from build123d import *

# Parameters (mm, degrees)
SK_BODY_W                     = 46.51
SK_BODY_H                     = 11.1
BODY_DEPTH                    = 8.4
SK_FLANGE_EARS_W              = 4.8
SK_FLANGE_EARS_H              = 5.6
FLANGE_EARS_DEPTH             = 6
SK_NOSE_W                     = 46.51
SK_NOSE_H                     = 7
NOSE_DEPTH                    = 7.2
FLANGE_SCREW_HOLES_DEPTH      = 32.081232681
FLANGE_SCREW_HOLES_DEPTH_BACK = 32.081232681
SK_FLANGE_SCREW_HOLES_R       = 1.35
SK_WIRE_ENTRIES_W             = 2.6
SK_WIRE_ENTRIES_H             = 2.8
WIRE_ENTRIES_DEPTH            = 6
SK_CONTACT_OPENINGS_W         = 1.6
SK_CONTACT_OPENINGS_H         = 1.6
CONTACT_OPENINGS_DEPTH        = 6.2
SK_CLAMP_SCREW_HOLES_R        = 1.3
CLAMP_SCREW_HOLES_DEPTH       = 3


with BuildPart() as part:
    # SK Body → Body (new body)
    with BuildSketch(Plane.XY.offset(3)):
        with Locations((0, 1.45)):
            Rectangle(SK_BODY_W, SK_BODY_H)
    extrude(amount=BODY_DEPTH)

    # SK Flange ears → Flange ears (add)
    with BuildSketch(Plane.XY.offset(3)):
        with Locations((25.655, 0)):
            Rectangle(SK_FLANGE_EARS_W, SK_FLANGE_EARS_H)
        with Locations((-25.655, 0)):
            Rectangle(SK_FLANGE_EARS_W, SK_FLANGE_EARS_H)
    extrude(amount=FLANGE_EARS_DEPTH)

    # SK Nose → Nose (add)
    with BuildSketch(Plane.XY.offset(3)):
        with Locations((0, -0.6)):
            Rectangle(SK_NOSE_W, SK_NOSE_H)
    extrude(amount=-NOSE_DEPTH)

    # SK Flange screw holes → Flange screw holes (cut, two sides: drawn at the far end of the back side and taken through both)
    with BuildSketch(Plane.XY.offset(-FLANGE_SCREW_HOLES_DEPTH_BACK)):
        with Locations((-25.375, 0)):
            Circle(SK_FLANGE_SCREW_HOLES_R)
        with Locations((25.375, 0)):
            Circle(SK_FLANGE_SCREW_HOLES_R)
    extrude(amount=FLANGE_SCREW_HOLES_DEPTH + FLANGE_SCREW_HOLES_DEPTH_BACK, mode=Mode.SUBTRACT)

    # SK Wire entries → Wire entries (cut)
    with BuildSketch(Plane.XY.offset(11.4)):
        with Locations((-20.955, -2)):
            Rectangle(SK_WIRE_ENTRIES_W, SK_WIRE_ENTRIES_H)
        with Locations((-17.145, -2)):
            Rectangle(SK_WIRE_ENTRIES_W, SK_WIRE_ENTRIES_H)
        with Locations((-13.335, -2)):
            Rectangle(SK_WIRE_ENTRIES_W, SK_WIRE_ENTRIES_H)
        with Locations((-9.525, -2)):
            Rectangle(SK_WIRE_ENTRIES_W, SK_WIRE_ENTRIES_H)
        with Locations((-5.715, -2)):
            Rectangle(SK_WIRE_ENTRIES_W, SK_WIRE_ENTRIES_H)
        with Locations((-1.905, -2)):
            Rectangle(SK_WIRE_ENTRIES_W, SK_WIRE_ENTRIES_H)
        with Locations((1.905, -2)):
            Rectangle(SK_WIRE_ENTRIES_W, SK_WIRE_ENTRIES_H)
        with Locations((5.715, -2)):
            Rectangle(SK_WIRE_ENTRIES_W, SK_WIRE_ENTRIES_H)
        with Locations((9.525, -2)):
            Rectangle(SK_WIRE_ENTRIES_W, SK_WIRE_ENTRIES_H)
        with Locations((13.335, -2)):
            Rectangle(SK_WIRE_ENTRIES_W, SK_WIRE_ENTRIES_H)
        with Locations((17.145, -2)):
            Rectangle(SK_WIRE_ENTRIES_W, SK_WIRE_ENTRIES_H)
        with Locations((20.955, -2)):
            Rectangle(SK_WIRE_ENTRIES_W, SK_WIRE_ENTRIES_H)
    extrude(amount=-WIRE_ENTRIES_DEPTH, mode=Mode.SUBTRACT)

    # SK Contact openings → Contact openings (cut)
    with BuildSketch(Plane.XY.offset(-4.2)):
        with Locations((-20.955, -0.6)):
            Rectangle(SK_CONTACT_OPENINGS_W, SK_CONTACT_OPENINGS_H)
        with Locations((-17.145, -0.6)):
            Rectangle(SK_CONTACT_OPENINGS_W, SK_CONTACT_OPENINGS_H)
        with Locations((-13.335, -0.6)):
            Rectangle(SK_CONTACT_OPENINGS_W, SK_CONTACT_OPENINGS_H)
        with Locations((-9.525, -0.6)):
            Rectangle(SK_CONTACT_OPENINGS_W, SK_CONTACT_OPENINGS_H)
        with Locations((-5.715, -0.6)):
            Rectangle(SK_CONTACT_OPENINGS_W, SK_CONTACT_OPENINGS_H)
        with Locations((-1.905, -0.6)):
            Rectangle(SK_CONTACT_OPENINGS_W, SK_CONTACT_OPENINGS_H)
        with Locations((1.905, -0.6)):
            Rectangle(SK_CONTACT_OPENINGS_W, SK_CONTACT_OPENINGS_H)
        with Locations((5.715, -0.6)):
            Rectangle(SK_CONTACT_OPENINGS_W, SK_CONTACT_OPENINGS_H)
        with Locations((9.525, -0.6)):
            Rectangle(SK_CONTACT_OPENINGS_W, SK_CONTACT_OPENINGS_H)
        with Locations((13.335, -0.6)):
            Rectangle(SK_CONTACT_OPENINGS_W, SK_CONTACT_OPENINGS_H)
        with Locations((17.145, -0.6)):
            Rectangle(SK_CONTACT_OPENINGS_W, SK_CONTACT_OPENINGS_H)
        with Locations((20.955, -0.6)):
            Rectangle(SK_CONTACT_OPENINGS_W, SK_CONTACT_OPENINGS_H)
    extrude(amount=CONTACT_OPENINGS_DEPTH, mode=Mode.SUBTRACT)

    # SK Clamp screw holes → Clamp screw holes (cut)
    with BuildSketch(Plane(origin=(0, 7, 0), x_dir=(1, 0, 0), z_dir=(0, 1, 0))):
        with Locations(Location((-20.955, -7.2, 0), (0, 0, 270))):
            Circle(SK_CLAMP_SCREW_HOLES_R)
        with Locations(Location((-17.145, -7.2, 0), (0, 0, 270))):
            Circle(SK_CLAMP_SCREW_HOLES_R)
        with Locations(Location((-13.335, -7.2, 0), (0, 0, 270))):
            Circle(SK_CLAMP_SCREW_HOLES_R)
        with Locations(Location((-9.525, -7.2, 0), (0, 0, 270))):
            Circle(SK_CLAMP_SCREW_HOLES_R)
        with Locations(Location((-5.715, -7.2, 0), (0, 0, 270))):
            Circle(SK_CLAMP_SCREW_HOLES_R)
        with Locations(Location((-1.905, -7.2, 0), (0, 0, 270))):
            Circle(SK_CLAMP_SCREW_HOLES_R)
        with Locations(Location((1.905, -7.2, 0), (0, 0, 270))):
            Circle(SK_CLAMP_SCREW_HOLES_R)
        with Locations(Location((5.715, -7.2, 0), (0, 0, 270))):
            Circle(SK_CLAMP_SCREW_HOLES_R)
        with Locations(Location((9.525, -7.2, 0), (0, 0, 270))):
            Circle(SK_CLAMP_SCREW_HOLES_R)
        with Locations(Location((13.335, -7.2, 0), (0, 0, 270))):
            Circle(SK_CLAMP_SCREW_HOLES_R)
        with Locations(Location((17.145, -7.2, 0), (0, 0, 270))):
            Circle(SK_CLAMP_SCREW_HOLES_R)
        with Locations(Location((20.955, -7.2, 0), (0, 0, 270))):
            Circle(SK_CLAMP_SCREW_HOLES_R)
    extrude(amount=-CLAMP_SCREW_HOLES_DEPTH, mode=Mode.SUBTRACT)


solid = part.part
Input: part model. Units: mm. Frame: model coordinates. A direction names the side the tool comes from. Coordinates: 2 decimals unless noted, no trailing zeros. Order: outer loops, then holes, each group sorted by start corner. A loop starts at its lowest first (then second) coordinate and runs counter-clockwise, first axis right, second up.
1. Ray query, line 1 along X through (y, z) = (0, 6.8) (3 decimals); line 2 along Y through (x, z) = (6, -2.5); line 3 along Z through (x, y) = (1, -0.75). Return the intervals inside material, ascending.
Checked values:
line 1: x = -28.055 to -26.725, -24.025 to 24.025, 26.725 to 28.055
line 2: y = -4.1 to -1.4, 0.2 to 2.9
line 3: z = -4.2 to 5.4
2. Access query for faces 3 (the flat face through (10, -3.4, 8)), 4 (the flat face through (27, 1, 3)), 5 (the flat face through (-14.135, -1, -1)), 6 (the cylindrical face through (-14.6, 5.5, 6.9)). Directions: +Z, -Z, +X, -X, +Y, -Y. A direction counts if a zero-diameter tool reaches every point of the face in a straight line with its end or side. Return the directions, or none.
Checked values:
face 3: +Z
face 4: -Z, +X, +Y, -Y
face 5: -Z
face 6: +Y
3. Cut plane A-A, the plane x = 0. Return loops of the section in (y, z).
Checked values:
outline: (-4.1, -4.2) - (2.9, -4.2) - (2.9, 3) - (7, 3) - (7, 11.4) - (-4.1, 11.4) - close
4. Contact query for flat-ended pins moving along their axis: P1, Ø1, axis at y = 5.5, z = 6.5, coming from the -X side (3 decimals); P2, Ø1.3, axis at x = -13.5, z = -2, coming from the +Y side; P3, Ø0.8, axis at x = -6, z = 6.5, coming from the +Y side. Output: stop coordinate, or through.
Checked values:
P1: stops at x = -23.255
P2: stops at y = 2.9
P3: stops at y = 4
5. Cut plane B-B, the plane z = 9.5. Count the separate pieces of the cut face and the enclosed holes in it, plus the area to 3 significant figures.
Checked values:
separate pieces: 1
enclosed holes: 12
area: 429 mm2
6. Draft query along X for faces 1 (the flat face through (-21.755, -1, -1)), 2 (the flat face through (-26, 2.8, 6)). Return one class per face: +X half, -X half, draft (parallel to the pull), parting line (faces both ways), or undercut.
Checked values:
face 1: undercut
face 2: draft
